Solid Edge part; units mm, degrees
sketch "Sketch1" plane through (0, 0, 0) normal (0, -1, 0) x (1, 0, 0)
  line L0 (6.5, 3.7528) -> (0, 7.5056)
  line L1 (0, 7.5056) -> (-6.5, 3.7528)
  line L2 (-6.5, 3.7528) -> (-6.5, -3.7528)
  line L3 (-6.5, -3.7528) -> (0, -7.5056)
  line L4 (0, -7.5056) -> (6.5, -3.7528)
  line L5 (6.5, -3.7528) -> (6.5, 3.7528)
extrude "Protrusion1" add sketch "Sketch1" along normal mid plane 7.9
sketch "Sketch2" plane through (0, 0, 0) normal (1, 0, 0) x (0, 1, 0)
  line L0 (-3.95, 5.75) -> (-3.4796, 7.5056)
revolve "RevolvedCutout1" cut sketch "Sketch2" angle 360 about axis through (0, 0, 0) along (0, -1, 0) material side at (0, -3.7631, 6.6407)
mirror "Mirror1" about plane through (0, 0, 0) normal (0, -1, 0) of "RevolvedCutout1"
hole "孔_7" at (0, -3.95, 0) direction (0, 1, 0) diameter 6.647 end up to next start chamfer 0.8 start chamfer angle 60 end chamfer 0.8 end chamfer angle 60
properties part number "N2611-0312" material "铝 1060"
Design review of the part built by this model. Coordinates are the model's own, in mm. Give positions to 0.01 mm unless a question says otherwise; leave off trailing zeros. Write each loop counter-clockwise with the first axis right and the second up, starting at its lowest first coordinate (ties: lowest second). Pieces come first, ordered by that corner, then holes. Notation, with made-up numbers: M -31.75,-26.75 L -20.75,-26.75 A37 cw -20.75,9.25 Z; hole C 14.25,37.25 d5. An arc over 180 degrees is marked long. Answer as a JSON object with one key per item and string values. Group by question number.
1) We need section B-B (y = -0.25). Give the boundary of the cut face in (x, z), and give its area (3 significant figures).
2) Clearance check with flat-ended pins moving along their axes: pin 1 Ø1 at (x, z) = (0, 1.5) entering from +Y; pin 2 Ø7.5 at (x, z) = (0, 0) entering from +Y; pin 3 Ø3 at (x, y) = (2, -2.5) entering from -Z. State where each tip first meets the part, or that it passes through.
3) Mouldability with a two-part tool opening along Z and no side actions: class faces 1 (the face through (-3.3, 0.1, -5.6)), 2 (the face through (3.3, 0.1, 5.6)), 3 (the face through (-4, -3.95, -2)), 4 (the face through (-1.27, -0.05, -3.07)) as released by +Z, released by -Z, zero draft, split by the parting line, or undercut.
4) We need section A-A (z = 0). Give the boundary of the cut face in (x, y).
5) For line 1 along X through (y, z) = (0.75, 0); line 2 along Z through (x, y) = (-3, -1); line 3 along X through (y, z) = (2, 1), list the stretches that pass through material, from the lowest coordinate up.
Answer key:
{
 "1": {"outline": "M -6.5,-3.75 L 0,-7.51 L 6.5,-3.75 L 6.5,3.75 L 0,7.51 L -6.5,3.75 Z; hole C 0,0 d6.65", "area": "112 mm²"},
 "2": {"pin 1": "passes through", "pin 2": "stops at y = 3.73", "pin 3": "stops at z = -7.22"},
 "3": {"face 1": "released by -Z", "face 2": "released by +Z", "face 3": "zero draft", "face 4": "undercut"},
 "4": {"outline": "M -6.5,-3.75 L -5.75,-3.95 L -4.12,-3.95 L -3.32,-3.49 L -3.32,3.49 L -4.12,3.95 L -5.75,3.95 L -6.5,3.75 Z; M 3.32,-3.49 L 4.12,-3.95 L 5.75,-3.95 L 6.5,-3.75 L 6.5,3.75 L 5.75,3.95 L 4.12,3.95 L 3.32,3.49 Z"},
 "5": {"line 1": "x = -6.5 to -3.32, 3.32 to 6.5", "line 2": "z = -5.77 to -1.43, 1.43 to 5.77", "line 3": "x = -6.5 to -3.17, 3.17 to 6.5"}
}
